```python
from build123d import *

# Parameters (mm, degrees)
F2_SIZE = 0.8


# Not quite as in the source:
# - a feature of the source that left no trace in its solid (it failed there, or was rolled back) is left out


with BuildPart() as f1:
    # F0 (on Front) → F1 (revolve)
    with BuildSketch(Plane.XZ):
        with BuildLine():
            Line((5.85, 6), (5.85, 0))
            Line((5.85, 0), (9.5, 0))
            Line((9.5, 0), (9.5, 0.294127265))
            ThreePointArc((9.5, 0.294127265), (9.3843349974, 0.6139500436), (9.090853561, 0.7858036122))
            ThreePointArc((9.090853561, 0.7858036122), (7.248319194, 3), (9.090853561, 5.2141963878))
            ThreePointArc((9.090853561, 5.2141963878), (9.3843349974, 5.3860499564), (9.5, 5.705872735))
            Line((9.5, 5.705872735), (9.5, 6))
            Line((9.5, 6), (5.85, 6))
        make_face()
    revolve(axis=Axis((0, 0, 22.371660918), (0, 0, 1)))

    # F2
    f2_edges = [f1.edges().sort_by_distance(p)[0] for p in [
        (-5.85, 0, 0),
        (-5.85, 0, 6),
    ]]
    chamfer(f2_edges, length=F2_SIZE)


solid = f1.part
```
The listing builds one solid part. Answer for the finished solid, in the listing's coordinates (mm). Coordinates: 2 decimals unless noted, no trailing zeros. Order: outer loops, then holes, each group sorted by start corner. A loop starts at its lowest first (then second) coordinate and runs counter-clockwise, first axis right, second up. Notation, with made-up numbers: M 82,50.25 L 130,50.25 A34 cw 130,83.25 Z; hole C 41.25,25 d11. An arc over 180 degrees is marked long. Answer as a JSON object with one key per item and string values. Group by question number.
1. Section C-C on z = 2.05 is taken. Write down the section's boundary in (x, y).
2. Straight lines are drawn through the part: line 1 (Y direction, x = 0, z = 1.05); line 2 (Y direction, x = 0, z = 2.7); line 3 (Z direction, x = 5.5, y = 7.25). For each, find the intervals that lie inside material, in ascending order.
3. Section A-A on y = 0 is taken. Write down the section's boundary in (x, z), then the cut area to 3 significant figures.
4. Section D-D on z = 3.85 is taken. Write down the section's boundary in (x, y), then the cut area to 3 significant figures.
5. Determine the mould class of faces 1 (the cylindrical face through (-1.27, -5.71, 2.97)), 2 (the flat face through (2, 6.5, 6)) for opening direction Y: released by +Y, released by -Y, zero draft, split by the parting line, or undercut.
6. Flat-ended cylindrical pins translate along their axes: P1, Ø2, axis at y = -7, z = 5.5, coming from the -X side; P2, Ø3, axis at y = -2, z = 5.5, coming from the -X side. Find the tip coordinate at first contact, or state that the pin passes through.
Values follow:
{
 "1": {"outline": "C 0,0 d14.92; hole C 0,0 d11.7"},
 "2": {"line 1": "-8.37 to -5.85, 5.85 to 8.37", "line 2": "-7.27 to -5.85, 5.85 to 7.27", "line 3": "0 to 0.78, 5.22 to 6"},
 "3": {"outline": "M -9.5,0 L -6.65,0 L -5.85,0.8 L -5.85,5.2 L -6.65,6 L -9.5,6 L -9.5,5.71 A0.5 ccw -9.09,5.21 A2.25 cw -9.09,0.79 A0.5 ccw -9.5,0.29 Z; M 5.85,0.8 L 6.65,0 L 9.5,0 L 9.5,0.29 A0.5 ccw 9.09,0.79 A2.25 cw 9.09,5.21 A0.5 ccw 9.5,5.71 L 9.5,6 L 6.65,6 L 5.85,5.2 Z", "area": "26.4 mm2"},
 "4": {"outline": "C 0,0 d14.83; hole C 0,0 d11.7", "area": "65.2 mm2"},
 "5": {"face 1": "undercut", "face 2": "zero draft"},
 "6": {"P1": "x = -7.35", "P2": "x = -9.49"}
}
